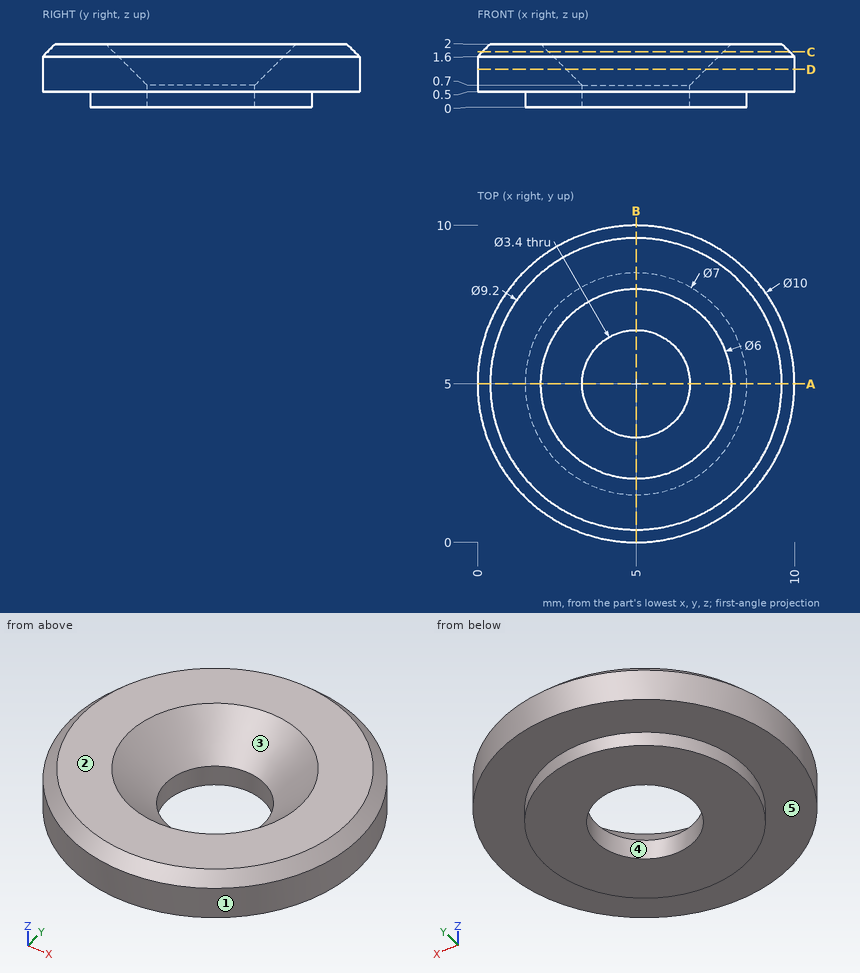
Job drawing, mm, ordinate dimensions from the low corner. One solid piece. A direction names the side the tool comes from. Coordinates: 2 decimals unless noted, no trailing zeros. Write each loop counter-clockwise with the first axis right and the second up, starting at its lowest first coordinate (ties: lowest second). Pieces come first, ordered by that corner, then holes. Notation, with made-up numbers: (9, 84.25) -> (62, 84.25) arc R20 cw to (62, 105.25) -> close; hole circle Ø7 at (78, -17). An arc over 180 degrees is marked (long way). Use CSV: the item, a comma, the result in double quotes. Start each with the question number.
Item 1: Band-saw the part on C-C, the plane z = 1.75. Write the cut outline in (x, y), plus the area to 3 significant figures.
Item 2: Wall check: probe 1 along Y at (x, z) = (5, 0.2); probe 2 along Z at (x, y) = (7, 1.75); probe 3 along Y at (x, z) = (5.75, 0.85). Give the ranges that are in metal, low to high.
Item 3: Tool access for the marked faces 4 and 5: list every direction of +Z, -Z, +X, -X, +Y, -Y with a clear straight run to the whole face (end or side of a thin tool).
Item 4: Drop a flat-ended pin along its axis: P1, Ø2.5, axis at x = 5, y = 5, coming from the +Z side. Give the stop position or say it passes through.
Item 5: Band-saw the part on A-A, the plane y = 5. Write the cut outline in (x, z), plus the area to 3 significant figures.
Item 6: Two-plate mould, pull along Y, no slides. Class the marked faces 1, 2 and 3: +Y half, -Y half, draft (parallel to the pull), parting line (faces both ways), or undercut.
Item 7: Band-saw the part on D-D, the plane z = 1.2. Write the cut outline in (x, y), plus the area to 3 significant figures.
Response values:
1,outline,"circle Ø9.7 at (5, 5); hole circle Ø5.5 at (5, 5)"
1,area,"50.1 mm2"
2,probe 1,"y = 1.5 to 3.3, 6.7 to 8.5"
2,probe 2,"z = 0.5 to 2"
2,probe 3,"y = 0.06 to 3.31, 6.69 to 9.94"
3,face 4,"+Z, -Z"
3,face 5,"-Z"
4,P1,"passes through"
5,outline,"(0, 0.5) -> (1.5, 0.5) -> (1.5, 0) -> (3.3, 0) -> (3.3, 0.7) -> (2, 2) -> (0.4, 2) -> (0, 1.6) -> close; (6.7, 0) -> (8.5, 0) -> (8.5, 0.5) -> (10, 0.5) -> (10, 1.6) -> (9.6, 2) -> (8, 2) -> (6.7, 0.7) -> close"
5,area,"9.85 mm2"
6,face 1,"parting line"
6,face 2,"draft"
6,face 3,"undercut"
7,outline,"circle Ø10 at (5, 5); hole circle Ø4.4 at (5, 5)"
7,area,"63.3 mm2"
